from build123d import *

# Parameters (mm, degrees)
SKETCH_4_W          = 196
SKETCH_4_H          = 1495.709506603
EXTRUDE_2_DEPTH     = 40
SKETCH_10_W         = 18.18
SKETCH_10_H         = 64.044231727
CUT_EXTRUDE_1_DEPTH = 46.474040195


with BuildPart() as part:
    # 草圖4 → 填料-伸長2 (new body)
    with BuildSketch(Plane(origin=(0, 40, 0), x_dir=(-1, 0, 0), z_dir=(0, 1, 0))):
        with Locations((0, 2.145246698)):
            Rectangle(SKETCH_4_W, SKETCH_4_H)
    extrude(amount=-EXTRUDE_2_DEPTH)

    # 草圖10 → 除料-伸長1 (cut, along a direction that is not the sketch's normal)
    with BuildSketch(Plane(origin=(0, 0, 0), x_dir=(1, 0, 0), z_dir=(0, 1, 0))):
        with Locations((42.342503168, -576.7595183)):
            Rectangle(SKETCH_10_W, SKETCH_10_H)
    extrude(amount=CUT_EXTRUDE_1_DEPTH, dir=(-0.13916051909627253, 0.9277367939751496, -0.34632180270604807), mode=Mode.SUBTRACT)


solid = part.part
Work out the finished part from the listing and answer in its coordinate system (mm). A direction names the side the tool comes from. Give positions to 0.01 mm unless a question says otherwise; leave off trailing zeros.
Q1. For a pull along X with two mould halves and no side action, classify faces 3 (the face through (1, 40, 13)), 4 (the face through (48.475, 19.72, 569.846)), 5 (the face through (39.17, 19.72, 601.42)), 6 (the face through (98, 20, -8)) as released by +X, released by -X, zero draft, split by the parting line, or undercut.
Answer:
face 3: zero draft
face 4: undercut
face 5: undercut
face 6: released by +X
Q2. Straight lines are drawn through the part: L1, parallel to X at y = 27, z = 594.5; L2, parallel to Z at x = 43, y = 11. For each, find the intervals that lie inside material, in ascending order.
Answer:
L1: x = -98 to 29.2, 47.38 to 98
L2: z = -745.71 to 540.63, 604.68 to 750
Q3. A tool of negligible diameter and unlimited length cuts with its end or side. For faces 1 (the face through (1, 20, 750)), 2 (the face through (39.173, 19.72, 537.376)), from which of +Z, -Z, +X, -X, +Y, -Y can it reach the whole face along a straight path? Write none if from no direction.
Answer:
face 1: +Z, +X, -X, +Y, -Y
face 2: none
